The model under review builds one solid part; all positions refer to its coordinate system, in mm. A direction names the side the tool comes from. Coordinates: 2 decimals unless noted, no trailing zeros. Write each loop counter-clockwise with the first axis right and the second up, starting at its lowest first coordinate (ties: lowest second). Pieces come first, ordered by that corner, then holes.
1) For line 1 (Z direction, x = 0, y = -1.2); line 2 (Z direction, x = 0, y = -2.2); line 3 (X direction, y = -1.1, z = -29), list the stretches that pass through material, from the lowest coordinate up.
2) Add section C-C, the plane y = -2.1. Give the number of separate pieces and of enclosed holes in the cut face, then the cut area to 3 significant figures.
3) Mouldability with a two-part tool opening along X and no side actions: class faces 3 (the cylindrical face through (-0.62, -1.5, -27.03)), 4 (the flat face through (4.762, -2, 0)), 5 (the cylindrical face through (-0.51, -2.196, -55.311)), 6 (the cylindrical face through (34.6, -2.2, -0.8)) as released by +X, released by -X, zero draft, split by the parting line, or undercut.
4) For P1, Ø1.5, axis at y = -1.5, z = -4.5, coming from the +X side, flat-tipped, find the tip position at first contact; note if it passes through.
5) Add section A-A, the plane z = 10. State the section outline as (x, y) points.
6) Add section D-D, the plane z = -41.5. State the section outline as (x, y) points.
7) Machinability: for faces 1 (the flat face through (-8, -3.048, 1)), 2 (the flat face through (-4.762, -2, 0)), which of the approach directions +Z, -Z, +X, -X, +Y, -Y give a long, thin tool a straight path to every point of the face, cutting with its end or side? Answer none if there is none.
8) Add section B-B, the plane x = 0. State the section outline as (y, z) points, then the cut area to 3 significant figures.
from build123d import *

# Parameters (mm, degrees)
F0_W        = 72.898
F0_H        = 114.3
F0_R        = 4.7625
F0_W_2      = 9.525
F0_H_2      = 25.4
F1_DEPTH    = 3.048
F2_T1_DEPTH = 96.1774845304
F2_T3_DEPTH = 137.5794845304


# Not quite as in the source:
# - a fillet or chamfer that OpenCascade refuses, or shapes differently, is made with other operations: its cross-section is extruded or revolved along the edge and cut away or added


with BuildPart() as f1:
    # F0 (on Front) → F1 (new body)
    with BuildSketch(Plane.XZ):
        Rectangle(F0_W, F0_H)
        with Locations((0, -31.75)):
            Circle(F0_R, mode=Mode.SUBTRACT)
        Rectangle(F0_W_2, F0_H_2, mode=Mode.SUBTRACT)
        with Locations((0, 31.75)):
            Circle(F0_R, mode=Mode.SUBTRACT)
    extrude(amount=F1_DEPTH)

    # F2: fillet of radius 5.08 on 4 edges, made by hand

    # F2_s2 → F2_t1 (cut)
    with BuildSketch(Plane.YZ.offset(-48.0887422652)):
        with BuildLine():
            ThreePointArc((0, 57.15), (-2.2182329348, 55.2765336861), (-3.048, 52.4941030939))
            Line((-3.048, 52.4941030939), (-3.048, 57.15))
            Line((-3.048, 57.15), (0, 57.15))
        make_face()
        with BuildLine():
            ThreePointArc((0, -57.15), (-2.2182329348, -55.2765336861), (-3.048, -52.4941030939))
            Line((-3.048, -52.4941030939), (-3.048, -57.15))
            Line((-3.048, -57.15), (0, -57.15))
        make_face()
    extrude(amount=F2_T1_DEPTH, mode=Mode.SUBTRACT)

    # F2_s4 → F2_t3 (cut)
    with BuildSketch(Plane.XY.offset(-68.7897422652)):
        with BuildLine():
            ThreePointArc((36.449, 0), (34.5755336861, -2.2182329348), (31.7931030939, -3.048))
            Line((31.7931030939, -3.048), (36.449, -3.048))
            Line((36.449, -3.048), (36.449, 0))
        make_face()
        with BuildLine():
            ThreePointArc((-36.449, 0), (-34.5755336861, -2.2182329348), (-31.7931030939, -3.048))
            Line((-31.7931030939, -3.048), (-36.449, -3.048))
            Line((-36.449, -3.048), (-36.449, 0))
        make_face()
    extrude(amount=F2_T3_DEPTH, mode=Mode.SUBTRACT)


solid = f1.part
Geometry results:
1. line 1: z = -56.41 to -36.51, -26.99 to -12.7, 12.7 to 26.99, 36.51 to 56.41
1. line 2: z = -55.3 to -36.51, -26.99 to -12.7, 12.7 to 26.99, 36.51 to 55.3
1. line 3: x = -35.79 to -3.89, 3.89 to 35.79
2. separate pieces: 1
2. enclosed holes: 3
2. area: 7,320 mm2
3. face 3: undercut
3. face 4: undercut
3. face 5: zero draft
3. face 6: released by +X
4. P1: stops at x = 36.04
5. outline: (-36.45, 0) arc R5.08 ccw to (-31.79, -3.05) - (-4.76, -3.05) - (-4.76, 0) - close; (4.76, -3.05) - (31.79, -3.05) arc R5.08 ccw to (36.45, 0) - (4.76, 0) - close
6. outline: (-36.45, 0) arc R5.08 ccw to (-31.79, -3.05) - (31.79, -3.05) arc R5.08 ccw to (36.45, 0) - close
7. face 1: +Z, -Z, +X, -X, -Y
7. face 2: +Y, -Y
8. outline: (-3.05, -52.49) arc R5.08 ccw to (0, -57.15) - (0, -36.51) - (-3.05, -36.51) - close; (-3.05, -26.99) - (0, -26.99) - (0, -12.7) - (-3.05, -12.7) - close; (-3.05, 12.7) - (0, 12.7) - (0, 26.99) - (-3.05, 26.99) - close; (-3.05, 36.51) - (0, 36.51) - (0, 57.15) arc R5.08 ccw to (-3.05, 52.49) - close
8. area: 205 mm2
